```python
from build123d import *

# Parameters (mm, degrees)
SKETCH3_W           = 19.05
SKETCH3_H           = 19.05
SKETCH3_W_2         = 15.875
SKETCH3_H_2         = 15.875
BOSS_EXTRUDE1_DEPTH = 222.25
FILLET1_R           = 0.79375
CUT_EXTRUDE1_REACH  = 225.268
CUT_EXTRUDE2_REACH  = 225.268
SKETCH5_W           = 15.875
SKETCH5_H           = 9.525
FILLET2_R           = 3.175
CUT_EXTRUDE3_DEPTH  = 224.268203345
SKETCH7_R           = 4.7625
SKETCH7_R_2         = 2.032
CUT_EXTRUDE4_DEPTH  = 224.268203458
CUT_EXTRUDE5_DEPTH  = 224.268203458


with BuildPart() as part:
    # Sketch3 → Boss-Extrude1 (new, symmetric)
    with BuildSketch(Plane.XY):
        Rectangle(SKETCH3_W, SKETCH3_H)
        Rectangle(SKETCH3_W_2, SKETCH3_H_2, mode=Mode.SUBTRACT)
    extrude(amount=BOSS_EXTRUDE1_DEPTH, both=True)

    # Fillet1
    fillet1_edges = [part.edges().sort_by_distance(p)[0] for p in [
        (9.525, -9.525, 0),
        (-9.525, -9.525, 0),
        (-9.525, 9.525, 0),
        (9.525, 9.525, 0),
    ]]
    fillet(fillet1_edges, radius=FILLET1_R)

    # Sketch4 → Cut-Extrude1 (cut, up to next)
    with BuildSketch(Plane(origin=(0, 9.525, 0), x_dir=(1, 0, 0), z_dir=(0, 1, 0)), mode=Mode.PRIVATE) as cut_extrude1_sk1:
        with BuildLine():
            Line((-3.96875, 209.55), (-3.96875, -222.25))
            Line((-3.96875, -222.25), (3.96875, -222.25))
            Line((3.96875, -222.25), (3.96875, 209.55))
            ThreePointArc((3.96875, 209.55), (0, 213.51875), (-3.96875, 209.55))
        make_face()
    cut_extrude1_tool1 = extrude(cut_extrude1_sk1.sketch, amount=-CUT_EXTRUDE1_REACH, mode=Mode.PRIVATE) & part.part
    add(cut_extrude1_tool1.solids().sort_by_distance((0, 9.525, 4.790573))[0], mode=Mode.SUBTRACT)

    # Sketch5 → Cut-Extrude2 (cut, up to next)
    with BuildSketch(Plane(origin=(0, -9.525, 0), x_dir=(-1, 0, 0), z_dir=(0, -1, 0)), mode=Mode.PRIVATE) as cut_extrude2_sk1:
        with Locations((0, -217.4875)):
            Rectangle(SKETCH5_W, SKETCH5_H)
    cut_extrude2_tool1 = extrude(cut_extrude2_sk1.sketch, amount=-CUT_EXTRUDE2_REACH, mode=Mode.PRIVATE) & part.part
    add(cut_extrude2_tool1.solids().sort_by_distance((0, -9.525, 217.4875))[0], mode=Mode.SUBTRACT)

    # Fillet2
    fillet2_edges = [part.edges().sort_by_distance(p)[0] for p in [
        (-7.9375, -8.73125, 212.725),
        (7.9375, -8.73125, 212.725),
    ]]
    fillet(fillet2_edges, radius=FILLET2_R)

    # Sketch6 → Cut-Extrude3 (cut, through all)
    with BuildSketch(Plane(origin=(9.525, 0, 0), x_dir=(0, 0, -1), z_dir=(1, 0, 0))):
        with BuildLine():
            Line((-222.25, -1.5875), (-222.25, -9.525))
            Line((-222.25, -9.525), (-214.3125, -9.525))
            ThreePointArc((-214.3125, -9.525), (-219.925160076, -7.200160076), (-222.25, -1.5875))
        make_face()
    extrude(amount=-CUT_EXTRUDE3_DEPTH, mode=Mode.SUBTRACT)

    # Sketch7 → Cut-Extrude4 (cut, through all)
    with BuildSketch(Plane(origin=(9.525, 0, 0), x_dir=(0, 0, -1), z_dir=(1, 0, 0))):
        with Locations((-214.3125, -1.5875)):
            Circle(SKETCH7_R)
        with Locations((215.9, 0)):
            Circle(SKETCH7_R_2)
    extrude(amount=-CUT_EXTRUDE4_DEPTH, mode=Mode.SUBTRACT)

    # Sketch8 → Cut-Extrude5 (cut, through all)
    with BuildSketch(Plane(origin=(9.525, 0, 0), x_dir=(0, 0, -1), z_dir=(1, 0, 0))):
        with BuildLine():
            Line((215.9, -9.525), (222.25, -9.525))
            Line((222.25, -9.525), (222.25, -3.175))
            ThreePointArc((222.25, -3.175), (220.390128061, -7.665128061), (215.9, -9.525))
        make_face()
    extrude(amount=-CUT_EXTRUDE5_DEPTH, mode=Mode.SUBTRACT)


solid = part.part
```
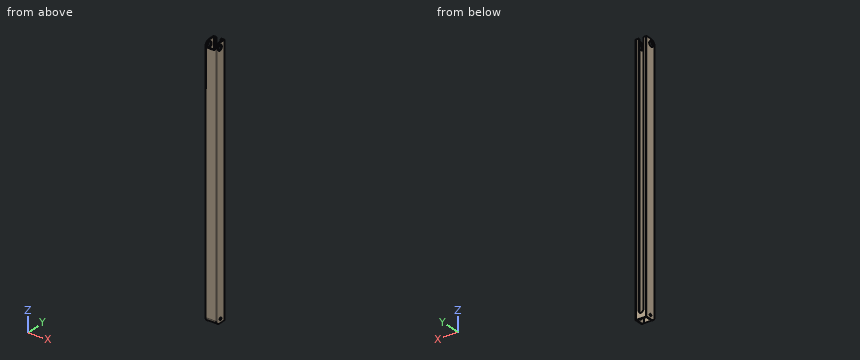
Design review of the part built by this model. Coordinates are the model's own, in mm. Coordinates: 2 decimals unless noted, no trailing zeros. Write each loop counter-clockwise with the first axis right and the second up, starting at its lowest first coordinate (ties: lowest second). Pieces come first, ordered by that corner, then holes.
1) Add section B-B (z = -66.5). Write out the cut boundary in (x, y) (1 decimal).
2) Insertion check: pin 1 (5.5 mm diameter, centred on y = 0, z = -215.9, fed in from +X) (3 decimals); pin 2 (0.8 mm diameter, centred on x = -0.5, y = -9, fed in from +Z) (3 decimals); pin 3 (8 mm diameter, centred on x = -1, y = -2, fed in from +Z). Each pin has a flat end and moves straight along its axis. Give the tip position at first contact, or say it passes through.
3) To check wall thickness, follow L1, parallel to X at y = -4.5, z = 174.5 (1 decimal); L2, parallel to Y at x = -8.45, z = -215.9 (3 decimals). State the ranges of each line that lie inside material, in increasing order.
Check result:
1. outline: (-9.5, -8.7) arc R0.8 ccw to (-8.7, -9.5) - (8.7, -9.5) arc R0.8 ccw to (9.5, -8.7) - (9.5, 8.7) arc R0.8 ccw to (8.7, 9.5) - (4, 9.5) - (4, 7.9) - (7.9, 7.9) - (7.9, -7.9) - (-7.9, -7.9) - (-7.9, 7.9) - (-4, 7.9) - (-4, 9.5) - (-8.7, 9.5) arc R0.8 ccw to (-9.5, 8.7) - close
2. pin 1: stops at x = 9.525
2. pin 2: stops at z = 212.725
2. pin 3: passes through
3. L1: x = -9.5 to -7.9, 7.9 to 9.5
3. L2: y = -9.525 to -2.032, 2.032 to 9.525
